Here's how the part is built. I have some questions about the finished solid (model axes, mm). Face numbers are marked on the shaded views. A direction names the side the tool comes from. Round coordinates to 2 decimals unless told otherwise and drop trailing zeros. Order: outer loops, then holes, each group sorted by start corner. A loop starts at its lowest first (then second) coordinate and runs counter-clockwise, first axis right, second up.
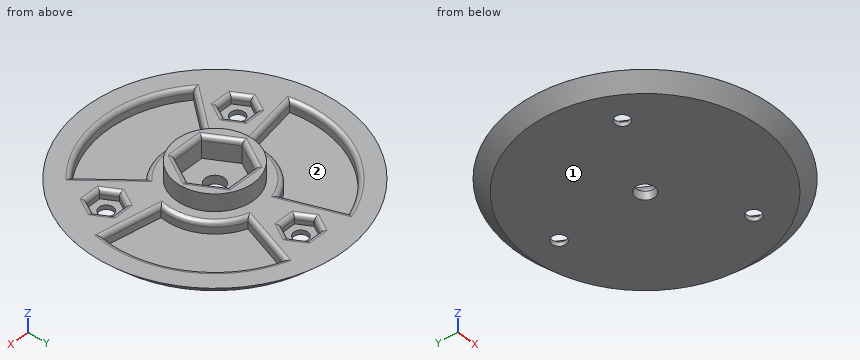
```python
from build123d import *

# Parameters (mm, degrees)
SKETCH004_R           = 30
SKETCH004_R_2         = 2.2
PAD001_DEPTH          = 3
POCKET004_DEPTH       = 2
POLARPATTERN002_COUNT = 3
POCKET002_DEPTH       = 2.6
POLARPATTERN004_COUNT = 3
SKETCH006_R           = 9
PAD_DEPTH             = 4
SKETCH007_R           = 1.625
POCKET_DEPTH          = 5
POLARPATTERN_COUNT    = 3
POCKET005_DEPTH       = 5
FILLET_R              = 1
CHAMFER_SIZE          = 2.99


with BuildPart() as part:
    # Sketch004 → Pad001 (new body)
    with BuildSketch(Plane.XY):
        Circle(SKETCH004_R)
        Circle(SKETCH004_R_2, mode=Mode.SUBTRACT)
    extrude(amount=PAD001_DEPTH)

    # Sketch005 (on Face4 of Pad001) → Pocket004 (cut)
    with BuildSketch(Plane.XY.offset(3)):
        Polygon((-1.75, 23.031089), (1.75, 23.031089), (3.5, 20), (1.75, 16.968911), (-1.75, 16.968911), (-3.5, 20), align=None)
    pocket004 = extrude(amount=-POCKET004_DEPTH, mode=Mode.SUBTRACT)

    # PolarPattern002: Pocket004 ×3 about axis
    polarpattern002_axis = Axis((0, 0, 3), (0, 0, 1))
    for i in range(1, POLARPATTERN002_COUNT):
        add(pocket004.rotate(polarpattern002_axis, i * 360 / POLARPATTERN002_COUNT), mode=Mode.SUBTRACT)

    # Sketch003 → Pocket002 (cut)
    with BuildSketch(Plane.XY.offset(3)):
        with BuildLine():
            ThreePointArc((-8.550504, 23.492316), (-21.650635, 12.5), (-24.620194, -4.341204))
            Line((-24.620194, -4.341204), (-11.817693, -2.083778))
            ThreePointArc((-4.104242, 11.276311), (-10.392305, 6), (-11.817693, -2.083778))
            Line((-8.550504, 23.492316), (-4.104242, 11.276311))
        make_face()
    pocket002 = extrude(amount=-POCKET002_DEPTH, mode=Mode.SUBTRACT)

    # PolarPattern004: Pocket002 ×3 about axis
    polarpattern004_axis = Axis((0, 0, 3), (0, 0, 1))
    for i in range(1, POLARPATTERN004_COUNT):
        add(pocket002.rotate(polarpattern004_axis, i * 360 / POLARPATTERN004_COUNT), mode=Mode.SUBTRACT)

    # Sketch006 → Pad (join)
    with BuildSketch(Plane.XY.offset(3)):
        Circle(SKETCH006_R)
    extrude(amount=PAD_DEPTH)

    # Sketch007 (on Face3 of PolarPattern002) → Pocket (cut)
    with BuildSketch(Plane.XY.offset(3)):
        with Locations((0, 20)):
            Circle(SKETCH007_R)
    pocket = extrude(amount=-POCKET_DEPTH, mode=Mode.SUBTRACT)

    # PolarPattern: Pocket ×3 about axis
    polarpattern_axis = Axis((0, 0, 3), (0, 0, 1))
    for i in range(1, POLARPATTERN_COUNT):
        add(pocket.rotate(polarpattern_axis, i * 360 / POLARPATTERN_COUNT), mode=Mode.SUBTRACT)

    # Sketch (on Face46 of PolarPattern) → Pocket005 (cut)
    with BuildSketch(Plane.XY.offset(7)):
        Polygon((-3.6, 6.235383), (3.6, 6.235383), (7.2, 0), (3.6, -6.235383), (-3.6, -6.235383), (-7.2, 0), align=None)
    extrude(amount=-POCKET005_DEPTH, mode=Mode.SUBTRACT)

    # Fillet
    fillet_edges = [part.edges().sort_by_distance(p)[0] for p in [
        (0, 23.031089, 3),
        (2.625, 21.515544, 3),
        (2.625, 18.484456, 3),
        (0, 16.968911, 3),
        (-2.625, 18.484456, 3),
        (-2.625, 21.515544, 3),
        (-6.327373, 17.384313, 3),
        (-21.650635, 12.5, 3),
        (-10.392305, 6, 3),
        (-18.218943, -3.212491, 3),
        (-17.320508, -6.968911, 3),
        (-19.945508, -8.484456, 3),
        (-14.695508, -8.484456, 3),
        (-14.695508, -11.515544, 3),
        (-17.320508, -13.031089, 3),
        (-19.945508, -11.515544, 3),
        (0, -12, 3),
        (-11.891571, -14.171822, 3),
        (11.891571, -14.171822, 3),
        (0, -25, 3),
        (17.320508, -6.968911, 3),
        (19.945508, -8.484456, 3),
        (19.945508, -11.515544, 3),
        (17.320508, -13.031089, 3),
        (14.695508, -11.515544, 3),
        (14.695508, -8.484456, 3),
        (18.218943, -3.212491, 3),
        (21.650635, 12.5, 3),
        (6.327373, 17.384313, 3),
        (10.392305, 6, 3),
        (0, 6.235383, 7),
        (5.4, 3.117691, 7),
        (5.4, -3.117691, 7),
        (0, -6.235383, 7),
        (-5.4, -3.117691, 7),
        (-5.4, 3.117691, 7),
    ]]
    fillet(fillet_edges, radius=FILLET_R)

    # Chamfer
    chamfer_edges = [part.edges().sort_by_distance(p)[0] for p in [
        (-30, 0, 0),
    ]]
    chamfer(chamfer_edges, length=CHAMFER_SIZE)


solid = part.part
```
1. If we section it at A-A, the plane z = 5.25: Write out the boundary of the cut face in (x, y).
Evaluation:
outline: circle Ø18 at (0, 0); hole (-7.2, 0) - (-3.6, -6.24) - (3.6, -6.24) - (7.2, 0) - (3.6, 6.24) - (-3.6, 6.24) - close
2. I need wall thicknesses on probe 1 along X at (y, z) = (13, 2.5); probe 2 along Y at (x, z) = (0, 0.5) (3 decimals); probe 3 along X at (y, z) = (22.5, 2.5). Which ranges of each line are inside material? Lowest first, please.
Evaluation:
probe 1: x = -26.49 to -21.51, -4.59 to 4.59, 21.51 to 26.49
probe 2: y = -27.51 to -25, -12 to -2.2, 2.2 to 18.375, 21.625 to 27.51
probe 3: x = -19.09 to -11.2, -8.05 to -2.21, 2.21 to 8.05, 11.2 to 19.09
3. If we section it at B-B, the plane x = 0: State how many separate pieces and enclosed holes the cut face has, and give its area (3 significant figures).
Evaluation:
separate pieces: 3
enclosed holes: 0
area: 121 mm2
4. I'm going to push flat-ended pins straight in: P1, Ø1, axis at x = -22.5, y = 13.5, coming from the +Z side; P2, Ø0.8, axis at x = -0.5, z = 1.5, coming from the +Y side; P3, Ø1.1, axis at x = 17, z = 1.5, coming from the +Y side. Where does each tip first touch, or does it pass through?
Evaluation:
P1: stops at z = 3
P2: stops at y = 28.91
P3: stops at y = 23.67
5. On a 3-axis mill with a long thin cutter (end or side, diameter ignored), from which of +Z, -Z, +X, -X, +Y, -Y can I reach the whole of each face in a straight line? I mean the marked faces 1 and 2. Say none if no direction works.
Evaluation:
face 1: -Z, +X, -X, +Y, -Y
face 2: +Z
